from build123d import *

# Parameters (mm, degrees)
F1_DEPTH = 2.54


with BuildPart() as f1:
    # F0 (on Front) → F1 (new body)
    with BuildSketch(Plane.XZ):
        with BuildLine():
            Line((403.098, 200.675558), (0, 200.675558))
            Line((0, 200.675558), (0, -151.876442))
            Line((0, -151.876442), (142.24, -151.876442))
            Line((142.24, -151.876442), (177.453318, -151.876442))
            ThreePointArc((177.453318, -151.876442), (299.929986, -122.086368), (403.098, -49.668528))
            Line((403.098, -49.668528), (403.098, -45.196442))
            Line((403.098, -45.196442), (403.098, 200.675558))
        make_face()
        Polygon((142.969289, -9.636442), (142.24, -149.334539), (3.269289, -149.336442), (3.269289, -9.636442), align=None, mode=Mode.SUBTRACT)
    extrude(amount=F1_DEPTH)


solid = f1.part
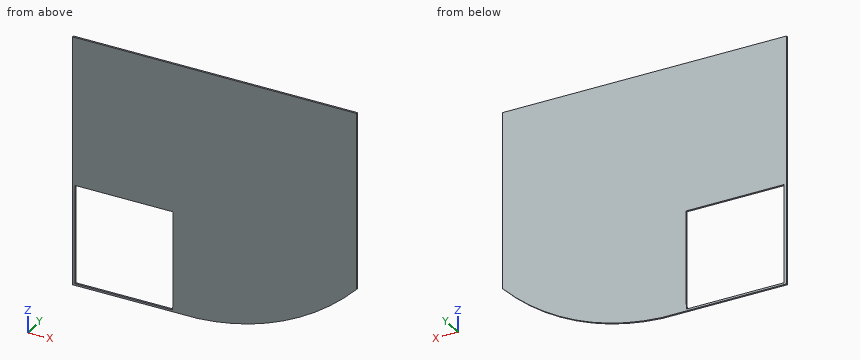
Input: part model. Units: mm. Frame: model coordinates. Give positions to 0.01 mm unless a question says otherwise; leave off trailing zeros. Loops run counter-clockwise (first coordinate to the right, second up) from the corner with the lowest first, then second, coordinate; pieces in that order, holes last. Notation, with made-up numbers: M 74.5,45 L 128.5,45 A21 ccw 128.5,68 Z; hole C 5.5,-10.5 d10. An arc over 180 degrees is marked long. Use CSV: the item, a comma, the result in double quotes.
(1) Pin query (flat end, axial travel): P1, Ø0.8, axis at y = -1, z = -66.5, coming from the +X side. Return the tip coordinate at first contact, or that it passes through.
Outcome:
P1,"stops at x = 385.94"
(2) Section A-A, the plane z = -62.5. Return loops of the section in (x, y).
Outcome:
outline,"M 0,-2.54 L 3.27,-2.54 L 3.27,0 L 0,0 Z; M 142.69,-2.54 L 389.91,-2.54 L 389.91,0 L 142.69,0 Z"
(3) Section D-D, the plane x = 352. Return loops of the section in (y, z), plus the area to 3 significant figures.
Outcome:
outline,"M -2.54,-92.72 L 0,-92.72 L 0,200.68 L -2.54,200.68 Z"
area,"745 mm²"
(4) Material intervals for L1, parallel to Z at x = 22.5, y = -1.5; L2, parallel to X at y = -1.8, z = -23.5; L3, parallel to Z at x = 201, y = -1.45, sorted ascending. Write a range as [from, to].
Outcome:
L1,"z = [-151.88, -149.34], [-9.64, 200.68]"
L2,"x = [0, 3.27], [142.9, 403.1]"
L3,"z = [-149.83, 200.68]"
(5) Section C-C, the plane x = 260. Return loops of the section in (y, z), plus the area to 3 significant figures.
Outcome:
outline,"M -2.54,-137.22 L 0,-137.22 L 0,200.68 L -2.54,200.68 Z"
area,"858 mm²"
(6) Section B-B, the plane y = -1.75. Return loops of the section in (x, z), plus the area to 3 significant figures.
Outcome:
outline,"M 0,-151.88 L 177.45,-151.88 A339.51 ccw 403.1,-49.67 L 403.1,200.68 L 0,200.68 Z; hole M 3.27,-149.34 L 142.24,-149.33 L 142.97,-9.64 L 3.27,-9.64 Z"
area,"115,000 mm²"
